from build123d import *

# Parameters (mm, degrees)
F1_W     = 5
F1_H     = 10
F1_R     = 1.6
F1_W_2   = 15
F1_H_2   = 5
F2_DEPTH = 5


with BuildPart() as f2:
    # F1 (on Front) → F2 (new body)
    with BuildSketch(Plane.XZ):
        with BuildLine():
            Line((-21, 35), (-21, 27))
            ThreePointArc((-21, 27), (-22.4644660941, 23.4644660941), (-26, 22))
            Line((-26, 22), (-26, 2))
            Line((-26, 2), (-46.0000009239, 2))
            Line((-46.0000009239, 2), (-46.0000009239, 22.0000018477))
            Line((-46.0000009239, 22.0000018477), (-51, 22.0000018477))
            Line((-51, 22.0000018477), (-51, -5))
            ThreePointArc((-51, -5), (-50.1213203436, -7.1213203436), (-48, -8))
            Line((-48, -8), (38, -8))
            ThreePointArc((38, -8), (40.1213203436, -7.1213203436), (41, -5))
            Line((41, -5), (41, 35))
            ThreePointArc((41, 35), (40.1213203436, 37.1213203436), (38, 38))
            Line((38, 38), (-18, 38))
            ThreePointArc((-18, 38), (-20.1213203436, 37.1213203436), (-21, 35))
        make_face()
        with Locations((-15.5, 0)):
            Rectangle(F1_W, F1_H, mode=Mode.SUBTRACT)
        with Locations((35.5, 0)):
            Rectangle(F1_W, F1_H, mode=Mode.SUBTRACT)
        with Locations((-15.5, 15)):
            Circle(F1_R, mode=Mode.SUBTRACT)
        with Locations((-15.5, 30)):
            Rectangle(F1_W, F1_H, mode=Mode.SUBTRACT)
        with Locations((10, 15)):
            Rectangle(F1_W_2, F1_H_2, mode=Mode.SUBTRACT)
        with Locations((35.5, 15)):
            Circle(F1_R, mode=Mode.SUBTRACT)
        with Locations((35.5, 30)):
            Rectangle(F1_W, F1_H, mode=Mode.SUBTRACT)
    extrude(amount=F2_DEPTH)


solid = f2.part
Model file for the job. Use its own axes, mm. A direction names the side the tool comes from. Give positions to 0.01 mm unless a question says otherwise; leave off trailing zeros. Write each loop counter-clockwise with the first axis right and the second up, starting at its lowest first coordinate (ties: lowest second). Pieces come first, ordered by that corner, then holes. Notation, with made-up numbers: (55.25, 19) -> (82.25, 19) arc R19 ccw to (82.25, 47) -> close; hole circle Ø1 at (24.5, -22.75). An arc over 180 degrees is marked (long way). Write item = value, one per line.
(1) Probe line 1 along X through (y, z) = (-1.25, 4); line 2 along Z through (x, y) = (35.5, -1.8); line 3 along Z through (x, y) = (37.5, -2.9). List the from-to ranges inside material, lowest first.
Determined:
line_1 = -51 to -46, -26 to -18, -13 to 33, 38 to 41
line_2 = -8 to -5, 5 to 13.4, 16.6 to 25, 35 to 38
line_3 = -8 to -5, 5 to 25, 35 to 38
(2) Slice it at C-C, the plane z = 19.5. Give the cut face in (x, y), then the cut area to 3 significant figures.
Determined:
outline = (-51, -5) -> (-46, -5) -> (-46, 0) -> (-51, 0) -> close; (-26, -5) -> (41, -5) -> (41, 0) -> (-26, 0) -> close
area = 360 mm2
(3) Flat gauge pin, fed straight in: P1, Ø2.5, axis at y = -3, z = 30, coming from the -X side. Where does the tip first touch, or does it go through?
Determined:
P1 = -21
(4) Tool access for faces 4 (the face through (35, -2, 35)), 5 (the face through (-48, -2, 22)), 6 (the face through (5, -5, 10)): list every direction of +Z, -Z, +X, -X, +Y, -Y with a clear straight run to the whole face (end or side of a thin tool).
Determined:
face_4 = +Y, -Y
face_5 = +Z, -X, +Y, -Y
face_6 = +Z, -Z, +X, -X, -Y
(5) Slice it at A-A, the plane z = 28. Give the cut face in (x, y).
Determined:
outline = (-21, -5) -> (-18, -5) -> (-18, 0) -> (-21, 0) -> close; (-13, -5) -> (33, -5) -> (33, 0) -> (-13, 0) -> close; (38, -5) -> (41, -5) -> (41, 0) -> (38, 0) -> close
(6) Slice it at D-D, the plane x = 4.5. Give the cut face in (y, z).
Determined:
outline = (-5, -8) -> (0, -8) -> (0, 12.5) -> (-5, 12.5) -> close; (-5, 17.5) -> (0, 17.5) -> (0, 38) -> (-5, 38) -> close
(7) Mould opens along Z. For faces 1 (the face through (-22, -2, 24)), 2 (the face through (-6, -2, -8)), 3 (the face through (38, -2, 30)) say: released by +Z, released by -Z, zero draft, split by the parting line, or undercut.
Determined:
face_1 = released by +Z
face_2 = released by -Z
face_3 = undercut
(8) Slice it at B-B, the plane x = 35.5. Give the cut face in (y, z).
Determined:
outline = (-5, -8) -> (0, -8) -> (0, -5) -> (-5, -5) -> close; (-5, 5) -> (0, 5) -> (0, 13.4) -> (-5, 13.4) -> close; (-5, 16.6) -> (0, 16.6) -> (0, 25) -> (-5, 25) -> close; (-5, 35) -> (0, 35) -> (0, 38) -> (-5, 38) -> close
